For this review, take the finished solid that the model builds, in its own axes (mm). Face numbers are marked on the shaded views. Give positions to 0.01 mm unless a question says otherwise; leave off trailing zeros. Write each loop counter-clockwise with the first axis right and the second up, starting at its lowest first coordinate (ties: lowest second). Pieces come first, ordered by that corner, then holes.
1) Draft analysis for pull direction Y (two halves, no side actions). For the marked faces 1 and 2, state which applies: pulls with the +Y half, pulls with the -Y half, needs draft (parallel to the pull), parting line crosses it, or undercut.
2) We need section A-A on x = -2.5. Give the boundary of the cut face in (y, z).
3) Wall thickness on line 1 along Y through (x, z) = (2.5, 0.8): over which ranges is the line inside the solid? List them lowest first.
4) We need section C-C on z = 0.8. Give the boundary of the cut face in (x, y), and give its area (3 significant figures).
from build123d import *

# Parameters (mm, degrees)
SKETCH1_W           = 40
SKETCH1_H           = 40
SKETCH1_W_2         = 6.3
SKETCH1_H_2         = 6.3
BOSS_EXTRUDE1_DEPTH = 1
PCB_START           = 1
SKETCH1_3_W         = 6.3
SKETCH1_3_H         = 6.3
PCB_DEPTH           = 0.4


with BuildPart() as part:
    # Sketch1 → Boss-Extrude1 (new body)
    # profile 1 of 2: a face of its own
    with BuildSketch(Plane.XY):
        Rectangle(SKETCH1_W, SKETCH1_H)
        Rectangle(SKETCH1_W_2, SKETCH1_H_2, mode=Mode.SUBTRACT)
    # profile 2 of 2: a face of its own
    with BuildSketch(Plane.XY):
        Rectangle(SKETCH1_W_2, SKETCH1_H_2)
    extrude(amount=BOSS_EXTRUDE1_DEPTH)

    # Sketch1<3> → PCB (cut)
    with BuildSketch(Plane.XY.offset(PCB_START)):
        Rectangle(SKETCH1_3_W, SKETCH1_3_H)
    extrude(amount=-PCB_DEPTH, mode=Mode.SUBTRACT)


solid = part.part
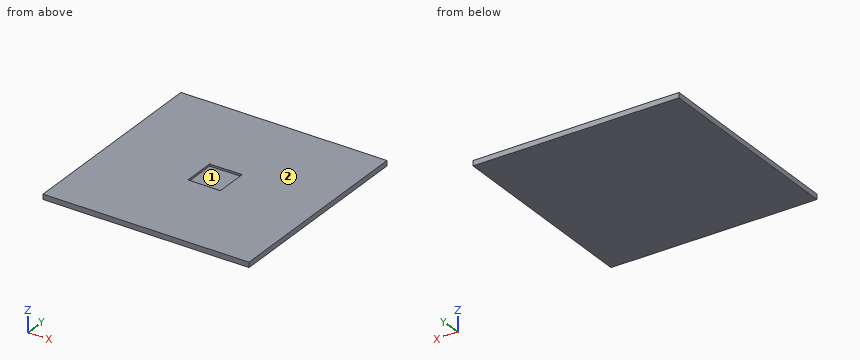
Results list:
1. face 1: undercut
1. face 2: needs draft
2. outline: (-20, 0) - (20, 0) - (20, 1) - (3.15, 1) - (3.15, 0.6) - (-3.15, 0.6) - (-3.15, 1) - (-20, 1) - close
3. line 1: y = -20 to -3.15, 3.15 to 20
4. outline: (-20, -20) - (20, -20) - (20, 20) - (-20, 20) - close; hole (-3.15, -3.15) - (3.15, -3.15) - (3.15, 3.15) - (-3.15, 3.15) - close
4. area: 1,560 mm2
